from build123d import *

# Parameters (mm, degrees)
SKETCH1_R           = 1.5
SKETCH1_W           = 52
SKETCH1_H           = 17
BOSS_EXTRUDE1_DEPTH = 3
BOSS_EXTRUDE2_DEPTH = 1
BOSS_EXTRUDE3_DEPTH = 2.822688649
FILLET1_R           = 20
FILLET3_R           = 5
SKETCH6_W           = 45.5
SKETCH6_H           = 2.072688649
CUT_EXTRUDE1_DEPTH  = 3
CHAMFER2_SIZE       = 20
CHAMFER2_SIZE_2     = 2.455691218


with BuildPart() as part:
    # Sketch1 → Boss-Extrude1 (new body)
    with BuildSketch(Plane.XY):
        with BuildLine():
            Line((-33.5, 56.672688649), (-43.5, 56.672688649))
            Line((-43.5, 56.672688649), (-43.5, 35.672688649))
            Line((-43.5, 35.672688649), (-59.995312317, 35.672688649))
            ThreePointArc((-59.995312317, 35.672688649), (-59.999578012, 34.697658936), (-59.9879988, 33.722688649))
            ThreePointArc((-59.9879988, 33.722688649), (0, -25.077311351), (59.9879988, 33.722688649))
            ThreePointArc((59.9879988, 33.722688649), (59.999578012, 34.697658936), (59.995312317, 35.672688649))
            Line((59.995312317, 35.672688649), (12, 35.672688649))
            Line((12, 35.672688649), (-33.5, 35.672688649))
            Line((-33.5, 35.672688649), (-33.5, 56.672688649))
        make_face()
        with Locations((-33, 15.25)):
            Circle(SKETCH1_R, mode=Mode.SUBTRACT)
        with Locations((0, 15.25)):
            Rectangle(SKETCH1_W, SKETCH1_H, mode=Mode.SUBTRACT)
        with Locations((33, 15.25)):
            Circle(SKETCH1_R, mode=Mode.SUBTRACT)
        with Locations((-36.25, 38.6)):
            Circle(SKETCH1_R, mode=Mode.SUBTRACT)
        with Locations((-36.25, 53.6)):
            Circle(SKETCH1_R, mode=Mode.SUBTRACT)
    extrude(amount=BOSS_EXTRUDE1_DEPTH)

    # Sketch4 → Boss-Extrude2 (add)
    with BuildSketch(Plane(origin=(0, 31.85, 0), x_dir=(1, 0, 0), z_dir=(0, 1, 0))):
        with BuildLine():
            Line((-25.4, 59.162140351), (-44.9909991, 0))
            Line((-44.9909991, 0), (45.0090009, 0))
            Line((45.0090009, 0), (25.4, 59.162140351))
            ThreePointArc((25.4, 59.162140351), (0, 49.25), (-25.4, 59.162140351))
        make_face()
    extrude(amount=BOSS_EXTRUDE2_DEPTH)

    # Sketch5 → Boss-Extrude3 (add)
    with BuildSketch(Plane(origin=(0, 32.85, 0), x_dir=(1, 0, 0), z_dir=(0, 1, 0))):
        with BuildLine():
            Line((-34.667242442, 31.176334461), (-44.9909991, 0))
            Line((-44.9909991, 0), (-44.9909991, -3))
            Line((-44.9909991, -3), (45.0090009, -3))
            Line((45.0090009, -3), (45.0090009, 0))
            Line((45.0090009, 0), (34.674298778, 31.180736875))
            ThreePointArc((34.674298778, 31.180736875), (0.004158519, 21.250000132), (-34.667242442, 31.176334461))
        make_face()
    extrude(amount=BOSS_EXTRUDE3_DEPTH)

    # Fillet1
    # the kernel refuses this fillet: 20 mm, written as the material it adds along each edge
    with BuildSketch(Plane(origin=(-43.5, 35.672688649, 0), x_dir=(0, 1, 0), z_dir=(0, 0, 1))) as fillet1_piece_1:
        with BuildLine():
            CenterArc((19.69053489, 20), FILLET1_R, 190.092298101, 79.907701899)
            Line((0, 16.495312317), (-0.393810698, 16.425218563))
            ThreePointArc((-0.393810698, 16.425218563), (-0.4, 8.247656158), (-0.4, 0))
            Line((-0.4, 0), (0, -0.4))
            Line((0, -0.4), (19.69053489, -0.4))
            Line((19.69053489, -0.4), (19.69053489, 0))
        make_face()
    extrude(amount=3)

    # Fillet3
    fillet3_edges = [part.edges().sort_by_distance(p)[0] for p in [
        (59.995312317, 35.672688649, 1.5),
        (-43.5, 56.672688649, 1.5),
        (-59.995312317, 35.672688649, 1.5),
    ]]
    fillet(fillet3_edges, radius=FILLET3_R)

    # Sketch6 → Cut-Extrude1 (cut)
    with BuildSketch(Plane.XY.offset(3)):
        with Locations((-10.75, 34.636344325)):
            Rectangle(SKETCH6_W, SKETCH6_H)
    extrude(amount=-CUT_EXTRUDE1_DEPTH, mode=Mode.SUBTRACT)

    # Chamfer2
    # the kernel refuses this chamfer: 20, 2.455691218 mm, written as the material it takes off along each edge
    with BuildSketch(Plane(origin=(-33.5, 35.672688649, 0), x_dir=(0, 0.00468857506979093, -0.9999890085715016), z_dir=(1, 0, 0))) as chamfer2_piece_1_section:
        Polygon((CHAMFER2_SIZE * 0.999989008572, -CHAMFER2_SIZE * 0.00468857506979), (-CHAMFER2_SIZE_2 * 0.0046885750699, -CHAMFER2_SIZE_2 * 0.999989008595), (0, 0), align=None)
    chamfer2_piece_1 = extrude(amount=45.5, mode=Mode.PRIVATE)
    chamfer2_piece_1 = split(chamfer2_piece_1, bisect_by=Plane(origin=(-10.75, 33.6, -6.806954436), z_dir=(0, 1, 0)), keep=Keep.TOP, mode=Mode.PRIVATE)
    add(chamfer2_piece_1, mode=Mode.SUBTRACT)


solid = part.part
Design review of the part built by this model. Coordinates are the model's own, in mm. A direction names the side the tool comes from. Round coordinates to 2 decimals unless told otherwise and drop trailing zeros. Loops run counter-clockwise (first coordinate to the right, second up) from the corner with the lowest first, then second, coordinate; pieces in that order, holes last. Notation, with made-up numbers: (-36, 22) -> (-4, 22) arc R17 ccw to (-4, 28) -> close; hole circle Ø7 at (49.5, 56.25). An arc over 180 degrees is marked (long way). Use one line per item in the form item = value. Start each with the question number.
Q1. We need section D-D on x = -36.25. Give the boundary of the cut face in (y, z).
Q2. Draft analysis for pull direction Y (two halves, no side actions). For faces 4 (the face through (-1, 31.85, -23)), 5 (the face through (-37.36, 39.61, 1.48)), 6 (the face through (0.516, 34.242, -21.252)), state which applies: +Y half, -Y half, draft (parallel to the pull), parting line (faces both ways), or undercut.
Q3. Machinability: for faces 1 (the face through (0, 23.75, 1)), 2 (the face through (-33.5, 43, 1)), 3 (the face through (15, 35.673, -11)), which of the approach directions +Z, -Z, +X, -X, +Y, -Y give a long, thin tool a straight path to every point of the face, cutting with its end or side? Answer none if there is none.
Q4. We need section C-C on z = -11.5. Give the boundary of the cut face in (x, y), then the cut area to 3 significant figures.
Q5. Wall thickness on line 1 along Y through (x, z) = (-36, 1); line 2 along Y through (x, z) = (-36.25, 1.05); line 3 along Y through (x, z) = (22, -25.5): over which ranges is each line inside the solid? List them lowest first. Write a range as [from, to].
Q6. We need section B-B on y = 19. Give the boundary of the cut face in (x, z), then the cut area to 3 significant figures.
Q7. For pin 1 Ø10 at (x, y) = (-4, -12.5) entering from -Z; pin 2 Ø11.5 at (y, z) = (44, -11.5) entering from +X; pin 3 Ø2.5 at (y, z) = (13, 1) entering from -X; pin 4 Ø0.6 at (y, z) = (35, -6.5) entering from -X, all flat-tipped, find the tip position at first contact; note any pin that passes through.
Q8. We need section A-A on x = 0. Give the boundary of the cut face in (y, z).
Calculated:
q1.outline = (-12.89, 0) -> (31.85, 0) -> (31.85, -26.4) -> (35.67, -26.4) -> (35.67, 0) -> (37.1, 0) -> (37.1, 3) -> (-12.89, 3) -> close; (40.1, 0) -> (52.1, 0) -> (52.1, 3) -> (40.1, 3) -> close; (55.1, 0) -> (56.67, 0) -> (56.67, 3) -> (55.1, 3) -> close
q2.face_4 = -Y half
q2.face_5 = undercut
q2.face_6 = draft
q3.face_1 = +Z, -Z
q3.face_2 = +Z, +Y
q3.face_3 = -Z, +X, +Y
q4.outline = (-41.18, 31.85) -> (41.2, 31.85) -> (41.2, 35.67) -> (12, 35.67) -> (12, 34.63) -> (-33.5, 34.63) -> (-33.5, 35.67) -> (-41.18, 35.67) -> close
q4.area = 267 mm²
q5.line_1 = [-13.08, 37.12], [40.08, 52.12], [55.08, 56.67]
q5.line_2 = [-12.89, 37.1], [40.1, 52.1], [55.1, 56.67]
q5.line_3 = [31.85, 32.85]
q6.outline = (-57.85, 0) -> (-26, 0) -> (-26, 3) -> (-57.85, 3) -> close; (26, 0) -> (57.85, 0) -> (57.85, 3) -> (26, 3) -> close
q6.area = 191 mm²
q7.pin_1 = 0
q7.pin_2 = through
q7.pin_3 = -56.33
q7.pin_4 = -42.94
q8.outline = (-25.08, 0) -> (6.75, 0) -> (6.75, 3) -> (-25.08, 3) -> close; (23.75, 0) -> (31.85, 0) -> (31.85, -49.25) -> (32.85, -49.25) -> (32.85, -21.25) -> (35.67, -21.25) -> (35.67, -20) -> (33.6, -3.12) -> (33.6, 3) -> (23.75, 3) -> close
